Could you check a few things on this model? Use its own coordinates, in mm. A direction names the side the tool comes from. Give positions to 0.01 mm unless a question says otherwise; leave off trailing zeros. Loops run counter-clockwise (first coordinate to the right, second up) from the corner with the lowest first, then second, coordinate; pieces in that order, holes last. Notation, with made-up numbers: (80, 77.5) - (124, 77.5) arc R17 ccw to (124, 94.5) - close; hole circle Ø11 at (59.25, -31.5). An arc over 180 degrees is marked (long way). Write each question's results on one line, items separated by ' | '. Start each with the question number.
(1) Suppose I cut it at B-B (z = 0). Please give me the cut outline in (x, y).
(2) For pin 1 (7 mm diameter, centred on x = -23.5, z = 22.5, fed in from +Y); pin 2 (1.5 mm diameter, centred on y = 2.5, z = 19, fed in from +X); pin 3 (2 mm diameter, centred on x = -15.5, y = 1, fed in from +Z); pin 4 (3 mm diameter, centred on x = -22.98, z = 22.98, fed in from -Y), each with a flat end and sliding along its axis, tell me the tip position at first contact or that it passes through.
(3) I need wall thicknesses on line 1 (Z direction, x = -11, y = 5.25); line 2 (Y direction, x = 20, z = 2.5); line 3 (Z direction, x = -15, y = 4.25). Which ranges of each line are inside material? Lowest first, please.
(4) If we mould it in two halves opening along X, with no side actions, what happens to faces 1 (the face through (7.43, 4.58, 17.94)), 2 (the face through (-26.556, 2.958, 26.477)), 3 (the face through (18.087, 4.584, 7.492))? For each: released by +X, released by -X, zero draft, split by the parting line, or undercut.
(5) Suppose I cut it at D-D (z = -15.5). Please give me the cut outline in (x, y), and give its area (3 significant figures).
(6) Suppose I cut it at A-A (x = 0). Please give me the cut outline in (y, z).
(7) On a 3-axis mill with a long thin cutter (end or side, diameter ignored), from which of +Z, -Z, +X, -X, +Y, -Y can I reach the whole of each face in a straight line? I mean faces 4 (the face through (0, 3, -19)), 5 (the face through (-19, 3, 0)), 6 (the face through (24.96, 4.52, -25.56)). Say none if no direction works.
(8) Suppose I cut it at C-C (y = 4.25). Count the separate pieces of the cut face and the enclosed holes in it, and give its area (3 significant figures).
from build123d import *

# Parameters (mm, degrees)
SKETCH1_R                      = 25
SKETCH1_R_2                    = 14
BOSS_EXTRUDE1_DEPTH            = 5
SKETCH3_R                      = 25
SKETCH3_R_2                    = 22.5
BOSS_EXTRUDE2_DEPTH            = 2
SKETCH5_R                      = 15.9
SKETCH5_R_2                    = 14
BOSS_EXTRUDE3_DEPTH            = 2
CUT_EXTRUDE1_DEPTH             = 4
CIRPATTERN1_COUNT              = 4
BOSS_EXTRUDE4_DEPTH            = 6
CBORE_FOR_M3_SHCS1_D           = 3.4
CBORE_FOR_M3_SHCS1_DEPTH       = 6
CBORE_FOR_M3_SHCS1_CBORE_D     = 6.5
CBORE_FOR_M3_SHCS1_CBORE_DEPTH = 3
FILLET1_R                      = 5
FILLET1_OF_MIRROR1_R           = 5
FILLET2_R                      = 1


with BuildPart() as part:
    # Sketch1 → Boss-Extrude1 (new body)
    with BuildSketch(Plane(origin=(0, 0, 0), x_dir=(1, 0, 0), z_dir=(0, 1, 0))):
        Circle(SKETCH1_R)
        Circle(SKETCH1_R_2, mode=Mode.SUBTRACT)
    extrude(amount=BOSS_EXTRUDE1_DEPTH)

    # Sketch3 → Boss-Extrude2 (add)
    with BuildSketch(Plane(origin=(0, 5, 0), x_dir=(1, 0, 0), z_dir=(0, 1, 0))):
        Circle(SKETCH3_R)
        Circle(SKETCH3_R_2, mode=Mode.SUBTRACT)
    extrude(amount=BOSS_EXTRUDE2_DEPTH)

    # Sketch5 → Boss-Extrude3 (add, through all)
    with BuildSketch(Plane(origin=(0, 5, 0), x_dir=(1, 0, 0), z_dir=(0, 1, 0))):
        Circle(SKETCH5_R)
        Circle(SKETCH5_R_2, mode=Mode.SUBTRACT)
    extrude(amount=BOSS_EXTRUDE3_DEPTH)

    # Sketch4 → Cut-Extrude1 (cut)
    with BuildSketch(Plane(origin=(0, 7, 0), x_dir=(1, 0, 0), z_dir=(0, 1, 0))):
        with BuildLine():
            Line((0, 0), (-9.567085809, 23.096988313))
            ThreePointArc((-9.567085809, 23.096988313), (0, 25), (9.567085809, 23.096988313))
            Line((9.567085809, 23.096988313), (0, 0))
        make_face()
    cut_extrude1 = extrude(amount=-CUT_EXTRUDE1_DEPTH, mode=Mode.SUBTRACT)

    # CirPattern1: Cut-Extrude1 ×4 about axis
    cirpattern1_axis = Axis((0, 7, 0), (0, -1, 0))
    for i in range(1, CIRPATTERN1_COUNT):
        add(cut_extrude1.rotate(cirpattern1_axis, i * 360 / CIRPATTERN1_COUNT), mode=Mode.SUBTRACT)

    # Sketch6 → Boss-Extrude4 (add)
    with BuildSketch(Plane.XZ):
        with BuildLine():
            Line((-30.0520382, 22.980970389), (-22.980970389, 30.0520382))
            Line((-22.980970389, 30.0520382), (-13.78497417, 20.856041982))
            ThreePointArc((-13.78497417, 20.856041982), (-17.67766953, 17.67766953), (-20.856041982, 13.78497417))
            Line((-20.856041982, 13.78497417), (-30.0520382, 22.980970389))
        make_face()
    boss_extrude4 = extrude(amount=-BOSS_EXTRUDE4_DEPTH)

    # CBORE for M3 SHCS1
    with Locations(Plane(origin=(0, 6, 0), x_dir=(1, 0, 0), z_dir=(0, 1, 0))):
        with Locations((-22.980970389, -22.980970389)):
            cbore_for_m3_shcs1 = CounterBoreHole(CBORE_FOR_M3_SHCS1_D / 2, CBORE_FOR_M3_SHCS1_CBORE_D / 2, CBORE_FOR_M3_SHCS1_CBORE_DEPTH, depth=CBORE_FOR_M3_SHCS1_DEPTH)

    # Fillet1
    fillet1_edges = [part.edges().sort_by_distance(p)[0] for p in [
        (-20.856041982, 3, 13.78497417),
        (-13.78497417, 3, 20.856041982),
    ]]
    fillet(fillet1_edges, radius=FILLET1_R)

    # Mirror1: Boss-Extrude4, CBORE for M3 SHCS1 across plane
    add(boss_extrude4.mirror(Plane(origin=(0, 0, 0), x_dir=(0.707106781, 0, 0.707106781), z_dir=(-0.707106781, 0, 0.707106781))))
    add(cbore_for_m3_shcs1.mirror(Plane(origin=(0, 0, 0), x_dir=(0.707106781, 0, 0.707106781), z_dir=(-0.707106781, 0, 0.707106781))), mode=Mode.SUBTRACT)

    # Fillet1 of Mirror1
    fillet1_of_mirror1_edges = [part.edges().sort_by_distance(p)[0] for p in [
        (13.78497417, 3, -20.856041982),
        (20.856041982, 3, -13.78497417),
    ]]
    fillet(fillet1_of_mirror1_edges, radius=FILLET1_OF_MIRROR1_R)

    # Fillet2
    fillet2_edges = [part.edges().sort_by_distance(p)[0] for p in [
        (-30.0520382, 3, 22.980970389),
        (-22.980970389, 3, 30.0520382),
        (22.980970389, 3, -30.0520382),
        (30.0520382, 3, -22.980970389),
    ]]
    fillet(fillet2_edges, radius=FILLET2_R)


solid = part.part
Output values:
1) outline: (-25, 0) - (-14, 0) - (-14, 3) - (-25, 3) - close; (14, 0) - (25, 0) - (25, 3) - (14, 3) - close
2) pin 1: y = 6 | pin 2: x = 17.09 | pin 3: z = 23.57 | pin 4: through
3) line 1: -22.45 to -19.63, -11.48 to -8.66, 8.66 to 11.48, 19.63 to 22.46 | line 2: 0 to 3 | line 3: -20 to -6.21, 6.21 to 22.52
4) face 1: undercut | face 2: released by -X | face 3: released by +X
5) outline: (-19.62, 0) - (22.78, 0) - (22.78, 6) - (19.62, 6) - (19.62, 7) - (16.31, 7) - (16.31, 5) - (6.42, 5) - (6.42, 3) - (-6.42, 3) - (-6.42, 5) - (-16.31, 5) - (-16.31, 7) - (-19.62, 7) - close | area: 203 mm2
6) outline: (0, -25) - (3, -25) - (3, -14) - (0, -14) - close; (0, 14) - (3, 14) - (3, 25) - (0, 25) - close
7) face 4: -Z, +Y | face 5: -X, +Y | face 6: +Y
8) separate pieces: 4 | enclosed holes: 2 | area: 870 mm2
